from build123d import *

# Parameters (mm, degrees)
SKETCH1_W                  = 25.5
SKETCH1_H                  = 75.5
MAIN_BODY_DEPTH            = 29
SKETCH2_W                  = 16
SKETCH2_H                  = 71.5
BATTERY_CUT_DEPTH          = 17
SKETCH3_W                  = 22
SKETCH3_H                  = 71.5
PCB_CUT_DEPTH              = 12
SKETCH4_W                  = 23.25
SKETCH4_H                  = 63.5
SOLAR_CUT_DEPTH            = 2
SKETCH5_W                  = 22
SKETCH5_H                  = 8.875
SOLAR_GAP_FILL_DEPTH       = 2
USB_CUT_DEPTH              = 2
USB_CLEARANCE_EMBOSS_DEPTH = 1
FILLET1_R                  = 2
SKETCH9_W                  = 23.5
SKETCH9_H                  = 73.5
SKETCH9_W_2                = 21.5
SKETCH9_H_2                = 71.5
CUT_EXTRUDE7_DEPTH         = 2
SKETCH10_W                 = 16
SKETCH10_H                 = 3
BOSS_EXTRUDE3_DEPTH        = 5
SKETCH11_W                 = 21.795239569
SKETCH11_H                 = 9.375
BOSS_EXTRUDE4_DEPTH        = 1


with BuildPart() as part:
    # Sketch1 → main body (new body)
    with BuildSketch(Plane.XY):
        with Locations((6.796111111, -10.402222222)):
            Rectangle(SKETCH1_W, SKETCH1_H)
    extrude(amount=MAIN_BODY_DEPTH)

    # Sketch2 → battery cut (cut)
    with BuildSketch(Plane.XY.offset(29)):
        with Locations((6.796111111, -10.402222222)):
            Rectangle(SKETCH2_W, SKETCH2_H)
    extrude(amount=-BATTERY_CUT_DEPTH, mode=Mode.SUBTRACT)

    # Sketch3 → pcb cut (cut)
    with BuildSketch(Plane(origin=(0, 0, 0), x_dir=(-1, 0, 0), z_dir=(0, 0, -1))):
        with Locations((-6.796111111, -10.402222222)):
            Rectangle(SKETCH3_W, SKETCH3_H)
    extrude(amount=-PCB_CUT_DEPTH, mode=Mode.SUBTRACT)

    # Sketch4 → solar cut (cut)
    with BuildSketch(Plane(origin=(0, 0, 0), x_dir=(-1, 0, 0), z_dir=(0, 0, -1))):
        with Locations((-6.796111111, -15.277222222)):
            Rectangle(SKETCH4_W, SKETCH4_H)
    extrude(amount=-SOLAR_CUT_DEPTH, mode=Mode.SUBTRACT)

    # Sketch6 → USB cut (cut)
    with BuildSketch(Plane.XZ.offset(48.152222222)):
        with BuildLine():
            Line((9.796111111, 5.5), (3.796111111, 5.5))
            ThreePointArc((3.796111111, 5.5), (2.046111111, 7.25), (3.796111111, 9))
            Line((3.796111111, 9), (9.796111111, 9))
            ThreePointArc((9.796111111, 9), (11.546111111, 7.25), (9.796111111, 5.5))
        make_face()
    extrude(amount=-USB_CUT_DEPTH, mode=Mode.SUBTRACT)

    # Sketch7 → USB clearance emboss (cut)
    with BuildSketch(Plane.XZ.offset(48.152222222)):
        with BuildLine():
            Line((9.296111111, 3.75), (4.296111111, 3.75))
            ThreePointArc((4.296111111, 3.75), (0.796111111, 7.25), (4.296111111, 10.75))
            Line((4.296111111, 10.75), (9.296111111, 10.75))
            ThreePointArc((9.296111111, 10.75), (12.796111111, 7.25), (9.296111111, 3.75))
        make_face()
    extrude(amount=-USB_CLEARANCE_EMBOSS_DEPTH, mode=Mode.SUBTRACT)

    # Fillet1
    fillet1_edges = [part.edges().sort_by_distance(p)[0] for p in [
        (-5.953888889, 27.347777778, 14.5),
        (19.546111111, 27.347777778, 14.5),
        (19.546111111, -48.152222222, 14.5),
        (-5.953888889, -48.152222222, 14.5),
    ]]
    fillet(fillet1_edges, radius=FILLET1_R)

    # Sketch9 → Cut-Extrude7 (cut)
    with BuildSketch(Plane.XY.offset(29)):
        with Locations((6.796111111, -10.402222222)):
            Rectangle(SKETCH9_W, SKETCH9_H)
        with Locations((6.796111111, -10.402222222)):
            Rectangle(SKETCH9_W_2, SKETCH9_H_2, mode=Mode.SUBTRACT)
    extrude(amount=-CUT_EXTRUDE7_DEPTH, mode=Mode.SUBTRACT)

    # Sketch10 → Boss-Extrude3 (add)
    with BuildSketch(Plane.XY.offset(29)):
        with Locations((6.796111111, 23.847777778)):
            Rectangle(SKETCH10_W, SKETCH10_H)
        with Locations((6.796111111, -44.652222222)):
            Rectangle(SKETCH10_W, SKETCH10_H)
    extrude(amount=-BOSS_EXTRUDE3_DEPTH)



with BuildPart() as body_2:
    # Sketch5 → solar gap fill (new body)
    with BuildSketch(Plane(origin=(0, 0, 0), x_dir=(-1, 0, 0), z_dir=(0, 0, -1))):
        with Locations((-6.796111111, 20.910277778)):
            Rectangle(SKETCH5_W, SKETCH5_H)
    extrude(amount=-SOLAR_GAP_FILL_DEPTH)


with BuildPart() as part_1:
    add(part.part)

    add(body_2.part)  # Boss-Extrude4 merges body 2
    # Sketch11 → Boss-Extrude4 (add)
    with BuildSketch(Plane.XY.offset(2)):
        with Locations((6.693730896, 20.660277778)):
            Rectangle(SKETCH11_W, SKETCH11_H)
    extrude(amount=BOSS_EXTRUDE4_DEPTH)


solid = part_1.part
Check sheet for the modelled part. Datum: model origin and axes. Units: mm. A direction names the side the tool comes from. Round coordinates to 2 decimals unless told otherwise and drop trailing zeros. Loops run counter-clockwise (first coordinate to the right, second up) from the corner with the lowest first, then second, coordinate; pieces in that order, holes last. Notation, with made-up numbers: (-21, 55) -> (1, 55) arc R14 ccw to (1, 82) -> close; hole circle Ø9 at (12.25, -19.5). An arc over 180 degrees is marked (long way). Put each result on its own line as item: value. Start each with the question number.
1. Section check B-B (z = 15.25). Enter the section's corners in (x, y).
2. Gauge pin test, flat ends, axial feed: pin 1 (3.5 mm diameter, centred on x = -3, y = -27, fed in from -Z); pin 2 (1.5 mm diameter, centred on x = 16, y = -25.5, fed in from -Z); pin 3 (1.5 mm diameter, centred on x = 5, y = 17, fed in from +Z). Record the tip position at first contact, or that the pin passes through.
3. Draft check along Y on faces 1 (the face through (-5.38, 26.75, 14.7)), 2 (the face through (7, -47.152, 28)), 3 (the face through (7, -47.152, 5)), 4 (the face through (-2, -13, 29)). Enter one of: +Y half, -Y half, draft (parallel to the pull), parting line (faces both ways), or undercut.
4. Section check D-D (z = 7.25). Enter the section's corners in (x, y), plus the area to 3 significant figures.
5. Section check C-C (y = 0.5). Enter the section's corners in (x, z).
6. Access from +Z, -Z, +X, -X, +Y, -Y to the whole of each face (thin tool, end or side, straight path). Record for faces 5 (the face through (17.546, -11, 28)), 6 (the face through (7, -45, 24)), 7 (the face through (7, 21, 3)), 8 (the face through (7, -48.152, 14)), 9 (the face through (11.546, -46.659, 7.288)).
7. Section check A-A (x = 7). Give the number of separate pieces and of enclosed holes in the cut face, plus the area to 3 significant figures.
8. Scan lines: probe 1 along X at (y, z) = (-40.5, 21.75); probe 2 along X at (y, z) = (19.5, 8.75); probe 3 along Y at (x, z) = (6, 19.5). Record each from-to range of solid material in increasing order.
Findings:
1. outline: (-5.95, -46.15) arc R2 ccw to (-3.95, -48.15) -> (17.55, -48.15) arc R2 ccw to (19.55, -46.15) -> (19.55, 25.35) arc R2 ccw to (17.55, 27.35) -> (-3.95, 27.35) arc R2 ccw to (-5.95, 25.35) -> close; hole (-1.2, -46.15) -> (14.8, -46.15) -> (14.8, 25.35) -> (-1.2, 25.35) -> close
2. pin 1: stops at z = 2
2. pin 2: stops at z = 12
2. pin 3: stops at z = 3
3. face 1: +Y half
3. face 2: undercut
3. face 3: -Y half
3. face 4: draft
4. outline: (-5.95, -46.15) arc R2 ccw to (-3.95, -48.15) -> (0.8, -48.15) -> (0.8, -47.15) -> (2.05, -47.15) -> (2.05, -46.15) -> (-4.2, -46.15) -> (-4.2, 25.35) -> (17.8, 25.35) -> (17.8, -46.15) -> (11.55, -46.15) -> (11.55, -47.15) -> (12.8, -47.15) -> (12.8, -48.15) -> (17.55, -48.15) arc R2 ccw to (19.55, -46.15) -> (19.55, 25.35) arc R2 ccw to (17.55, 27.35) -> (-3.95, 27.35) arc R2 ccw to (-5.95, 25.35) -> close
4. area: 327 mm^2
5. outline: (-5.95, 0) -> (-4.83, 0) -> (-4.83, 2) -> (-4.2, 2) -> (-4.2, 12) -> (-1.2, 12) -> (-1.2, 29) -> (-3.95, 29) -> (-3.95, 27) -> (-4.95, 27) -> (-4.95, 29) -> (-5.95, 29) -> close; (14.8, 12) -> (17.8, 12) -> (17.8, 2) -> (18.42, 2) -> (18.42, 0) -> (19.55, 0) -> (19.55, 29) -> (18.55, 29) -> (18.55, 27) -> (17.55, 27) -> (17.55, 29) -> (14.8, 29) -> close
6. face 5: +Z
6. face 6: -Z
6. face 7: none
6. face 8: +Z, -Z, +X, -X, -Y
6. face 9: -Y
7. separate pieces: 3
7. enclosed holes: 0
7. area: 157 mm^2
8. probe 1: x = -5.95 to -1.2, 14.8 to 19.55
8. probe 2: x = -5.95 to -4.2, 17.8 to 19.55
8. probe 3: y = -48.15 to -46.15, 25.35 to 27.35
